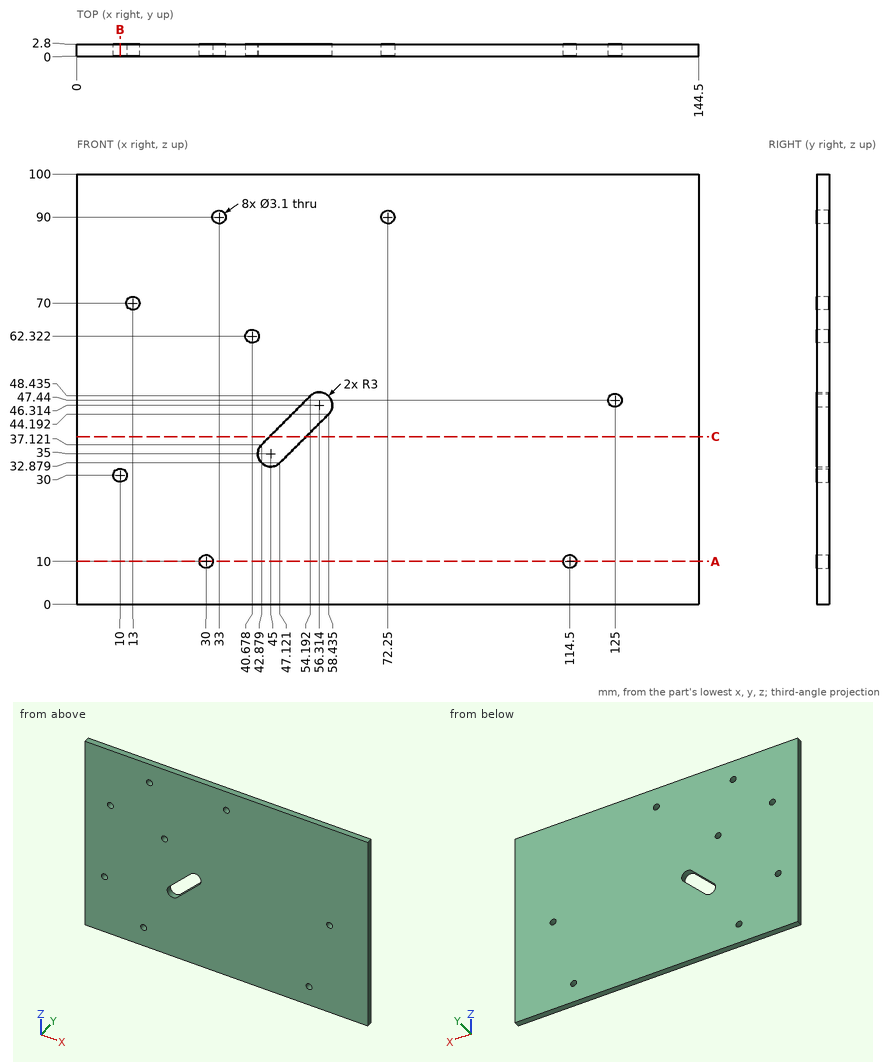
Check sheet for the drawn part. Datum: minimum x, y, z corner. Units: mm. Give positions to 0.01 mm unless a question says otherwise; leave off trailing zeros. Order: outer loops, then holes, each group sorted by start corner. A loop starts at its lowest first (then second) coordinate and runs counter-clockwise, first axis right, second up. Notation, with made-up numbers: (2.5, 62.25) - (14.5, 62.25) arc R28 ccw to (14.5, 83.25) - close; hole circle Ø3 at (33, 79.25). An arc over 180 degrees is marked (long way). Answer as a JSON object with one key per item and string values.
(1) Cross-section at C-C (z = 39). Record the cut outline in (x, y).
Report:
{"outline": "(0, 0) - (44.76, 0) - (44.76, 2.8) - (0, 2.8) - close; (53.24, 0) - (144.5, 0) - (144.5, 2.8) - (53.24, 2.8) - close"}
(2) Material ranges on line 1 (X direction, y = 0.8, z = 90); line 2 (Z direction, x = 125, y = 2.2); line 3 (Z direction, x = 10, y = 1.5), recorded low to high.
Report:
{"line 1": "0 to 31.45, 34.55 to 70.7, 73.8 to 144.5", "line 2": "0 to 45.89, 48.99 to 100", "line 3": "0 to 28.45, 31.55 to 100"}
(3) Depth check by flat-ended pin: pin 1 Ø1.5 at (x, z) = (51, 58) entering from -Y. Enter the tip coordinate at first touch or a pass-through.
Report:
{"pin 1": "y = 0"}
(4) Cross-section at A-A (z = 10). Record the cut outline in (x, y).
Report:
{"outline": "(0, 0) - (28.45, 0) - (28.45, 2.8) - (0, 2.8) - close; (31.55, 0) - (112.95, 0) - (112.95, 2.8) - (31.55, 2.8) - close; (116.05, 0) - (144.5, 0) - (144.5, 2.8) - (116.05, 2.8) - close"}
(5) Cross-section at B-B (x = 10). Record the cut outline in (y, z), then the cut area to 3 significant figures.
Report:
{"outline": "(0, 0) - (2.8, 0) - (2.8, 28.45) - (0, 28.45) - close; (0, 31.55) - (2.8, 31.55) - (2.8, 100) - (0, 100) - close", "area": "271 mm^2"}
